```python
from build123d import *

# Parameters (mm, degrees)
SKETCH1_R           = 63.5
SKETCH1_R_2         = 53.975
BOSS_EXTRUDE1_DEPTH = 12.7
SKETCH2_R           = 57.15
CUT_EXTRUDE1_DEPTH  = 1.5875
CUT_EXTRUDE2_START  = -1.5875
SKETCH3_R           = 57.15
CUT_EXTRUDE2_DEPTH  = 1.5875


with BuildPart() as part:
    # Sketch1 → Boss-Extrude1 (new, symmetric)
    with BuildSketch(Plane.XY):
        Circle(SKETCH1_R)
        Circle(SKETCH1_R_2, mode=Mode.SUBTRACT)
    extrude(amount=BOSS_EXTRUDE1_DEPTH, both=True)

    # Sketch2 → Cut-Extrude1 (cut)
    with BuildSketch(Plane.XY.offset(12.7)):
        Circle(SKETCH2_R)
    extrude(amount=-CUT_EXTRUDE1_DEPTH, mode=Mode.SUBTRACT)

    # Sketch3 → Cut-Extrude2 (cut)
    with BuildSketch(Plane(origin=(0, 0, -12.7), x_dir=(-1, 0, 0), z_dir=(0, 0, -1)).offset(CUT_EXTRUDE2_START)):
        with Locations(Location((0, 0, 0), (0, 0, 180))):
            Circle(SKETCH3_R)
    extrude(amount=CUT_EXTRUDE2_DEPTH, mode=Mode.SUBTRACT)


solid = part.part
```
Source: CAD feature listing. Evaluate the final solid. Frame: model axes, mm. A direction names the side the tool comes from. Round coordinates to 2 decimals unless told otherwise and drop trailing zeros. Loops run counter-clockwise (first coordinate to the right, second up) from the corner with the lowest first, then second, coordinate; pieces in that order, holes last.
(1) Section query C-C (z = -3.5). Output: boundary loops of the cut face in (x, y) (3 decimals), and give its area (3 significant figures).
From the geometry:
outline: circle Ø127 at (0, 0); hole circle Ø107.95 at (0, 0)
area: 3,520 mm2
(2) Material intervals for probe 1 along Y at (x, z) = (0, -11.45); probe 2 along X at (y, z) = (-1, -3.5); probe 3 along Y at (x, z) = (0, -10) (3 decimals), sorted ascending.
From the geometry:
probe 1: y = -63.5 to -57.15, 57.15 to 63.5
probe 2: x = -63.49 to -53.97, 53.97 to 63.49
probe 3: y = -63.5 to -53.975, 53.975 to 63.5
(3) Access query for faces 5 (the flat face through (42.1, -34.1, -11.112)), 6 (the flat face through (-57, 10, -12.7)), 7 (the flat face through (42.1, 34.1, 11.112)). Directions: +Z, -Z, +X, -X, +Y, -Y. A direction counts if a zero-diameter tool reaches every point of the face in a straight line with its end or side. Return the directions, or none.
From the geometry:
face 5: -Z
face 6: -Z, +X, -X, +Y, -Y
face 7: +Z
(4) Pull-direction query (Y, two-part tool) for faces 1 (the cylindrical face through (-57.095, 2.513, 11.917)), 2 (the flat face through (-57, 10, 12.7)), 3 (the cylindrical face through (-57.095, -2.513, -11.895)), 4 (the cylindrical face through (-13.77, -61.99, 0.18)); classes: +Y half, -Y half, draft (parallel to the pull), parting line (faces both ways), or undercut.
From the geometry:
face 1: undercut
face 2: draft
face 3: undercut
face 4: parting line
(5) Contact query for flat-ended pins moving along their axis: pin 1 Ø10 at (y, z) = (-3, -9.5) entering from -X; pin 2 Ø4 at (x, z) = (-10, -8) entering from -Y; pin 3 Ø12 at (y, z) = (20, 9.5) entering from +X; pin 4 Ø10 at (x, z) = (12, -2.5) entering from -Y. Output: stop coordinate, or through.
From the geometry:
pin 1: stops at x = -63.5
pin 2: stops at y = -62.99
pin 3: stops at x = 61.94
pin 4: stops at y = -63.11
